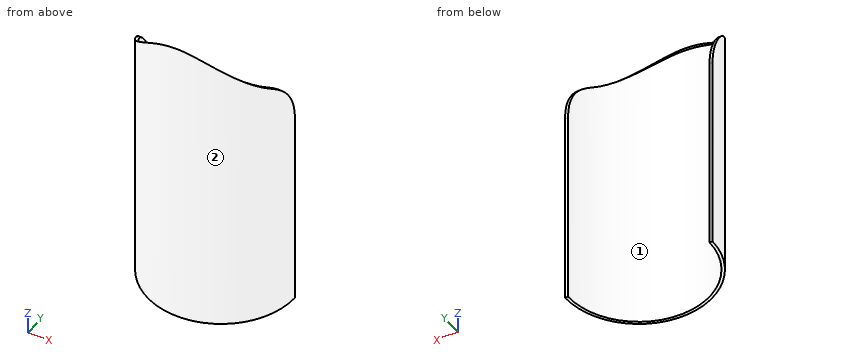
```python
from build123d import *

# Parameters (mm, degrees)
EXTRUDE_THIN1_DEPTH     = 200
CUT_EXTRUDE1_DEPTH      = 213.132034356
CUT_EXTRUDE1_DEPTH_BACK = 213.132034356
FILLET1_R               = 40


with BuildPart() as part:
    # Sketch1 → Extrude-Thin1 (new body)
    with BuildSketch(Plane.XY):
        with BuildLine():
            ThreePointArc((-50, 0), (0, -50), (50, 0))
            Line((50, 0), (48, 0))
            ThreePointArc((48, 0), (0, -48), (-48, 0))
            Line((-48, 0), (-50, 0))
        make_face()
    extrude(amount=-EXTRUDE_THIN1_DEPTH)

    # Sketch2 → Cut-Extrude1 (cut, two sides: drawn at the far end of the back side and taken through both)
    with BuildSketch(Plane(origin=(0, 0, 0), x_dir=(0, 0, -1), z_dir=(1, 0, 0)).offset(-CUT_EXTRUDE1_DEPTH_BACK)):
        with BuildLine():
            Line((0, 0), (0, -50))
            ThreePointArc((0, -50), (25.082111762, -29.065689409), (40, 0))
            Line((40, 0), (0, 0))
        make_face()
    extrude(amount=CUT_EXTRUDE1_DEPTH + CUT_EXTRUDE1_DEPTH_BACK, mode=Mode.SUBTRACT)

    # Fillet1
    # the kernel refuses this fillet: 40 mm, written as the material it takes off along each edge
    with BuildSketch(Plane(origin=(115.07027284, 0, -40), x_dir=(0, 0, -1), z_dir=(-1, 0, 0)), Plane(origin=(17.07027284, 0, -40), x_dir=(0, 0, -1), z_dir=(-1, 0, 0))) as fillet1_piece_1:
        with BuildLine():
            CenterArc((26.028109136, 40), FILLET1_R, 210.63069692, 59.36930308)
            ThreePointArc((-8.390657995, 19.619900167), (-3.554396204, 10.084051777), (0, 0))
            Line((0, 0), (26.028109136, 0))
        make_face()
    extrude(amount=132.140545681, mode=Mode.SUBTRACT)


solid = part.part
```
Model file for the job. Use its own axes, mm. Face numbers are marked on the shaded views. Round coordinates to 2 decimals unless told otherwise and drop trailing zeros. Loops run counter-clockwise (first coordinate to the right, second up) from the corner with the lowest first, then second, coordinate; pieces in that order, holes last. Notation, with made-up numbers: M -10.75,-32 L 11.25,-32 A15 cw 11.25,-14 Z; hole C 68.5,26 d9. An arc over 180 degrees is marked long. Put each result on its own line as item: value. Start each with the question number.
Item 1: Drop flat-ended pins along their axis: P1, Ø2, axis at y = -42.5, z = -78, coming from the -X side; P2, Ø5, axis at x = -36.5, y = -25.5, coming from the -Z side; P3, Ø8, axis at x = 37, z = -74.5, coming from the +Y side; P4, Ø8, axis at y = -22, z = -64.5, coming from the -X side. Give the stop position or say it passes through.
Item 2: Cut at B-B (z = -118). List the corners of the cut face in (x, y), then the cut area to 3 significant figures.
Item 3: Cut at C-C (y = -17.5). List the corners of the cut face in (x, z), then the cut area to 3 significant figures.
Item 4: Cut at D-D (x = 0). List the corners of the cut face in (y, z), then the cut area to 3 significant figures.
Item 5: Mould opens along X. For the marked faces 1 and 2 say: released by +X, released by -X, zero draft, split by the parting line, or undercut.
Item 6: Cut at A-A (y = -33). List the corners of the cut face in (x, z), then the cut area to 3 significant figures.
Item 7: Drill centre lines: line 1 along Y through (x, z) = (1, -152.5); line 2 along X through (y, z) = (-43, -93); line 3 along X through (y, z) = (-33.5, -52). Where is each one in solid material? Low to high.
Answer block:
1. P1: x = -27.89
1. P2: through
1. P3: y = -24.96
1. P4: x = -46.65
2. outline: M -50,0 A50 ccw 50,0 L 48,0 A48 cw -48,0 Z
2. area: 308 mm2
3. outline: M -46.84,-200 L -44.7,-200 L -44.7,-32.96 L -46.84,-32.96 Z; M 44.7,-200 L 46.84,-200 L 46.84,-32.96 L 44.7,-32.96 Z
3. area: 715 mm2
4. outline: M -50,-200 L -48,-200 L -48,-3.5 A82 cw -50,0 Z
4. area: 396 mm2
5. face 1: undercut
5. face 2: split by the parting line
6. outline: M -37.56,-200 L -34.86,-200 L -34.86,-21.73 L -37.56,-21.73 Z; M 34.86,-200 L 37.56,-200 L 37.56,-21.73 L 34.86,-21.73 Z
6. area: 965 mm2
7. line 1: -49.99 to -47.99
7. line 2: -25.51 to -21.33, 21.33 to 25.51
7. line 3: -37.12 to -34.38, 34.38 to 37.12
